Can you work these out from the model? Positions are in its coordinate system, mm. A direction names the side the tool comes from. Coordinates: 2 decimals unless noted, no trailing zeros. Order: outer loops, then holes, each group sorted by start corner. A loop starts at its lowest first (then second) coordinate and runs counter-clockwise, first axis right, second up. Notation, with made-up numbers: (-20, 87) -> (32, 87) arc R14 cw to (32, 107) -> close; hole circle Ø11 at (51.5, 18). An arc over 180 degrees is marked (long way). Write item = value, one per line. Start each with the question number.
from build123d import *

# Parameters (mm, degrees)
AXIAL_HOLES_DEPTH                            = 167.945530039
AXIAL_HOLES_DEPTH_BACK                       = 167.945530039
SKETCH2_R                                    = 2.3
SKETCH2_R_2                                  = 1.65
DRY_START                                    = 159.2
SKETCH3_W                                    = 1
SKETCH3_H                                    = 8.8
DRY_INTERFACE_VENT_NOT_A_COOLANT_PASSA_DEPTH = 0.5


with BuildPart() as part:
    # Axial profile (mm) → Full revolution (revolve)
    with BuildSketch(Plane.XY, mode=Mode.PRIVATE) as full_revolution_sk:
        Polygon((156.7, 0), (159.65, 0), (159.65, 26.2), (159.2, 26.2), (159.2, 27.2), (159.7, 27.2), (159.7, 34.4), (156.7, 34.4), align=None)
    revolve(full_revolution_sk.sketch.rotate(Axis((-110, 0, 0), (1, 0, 0)), 90), axis=Axis((-110, 0, 0), (1, 0, 0)))

    # Sketch2 → Axial holes (cut, two sides: drawn at the far end of the back side and taken through both)
    with BuildSketch(Plane(origin=(0, 0, 0), x_dir=(0, 0, -1), z_dir=(1, 0, 0)).offset(-AXIAL_HOLES_DEPTH_BACK)):
        with Locations(Location((-1.977382665, 12.848733704, 0), (0, 0, 180))):
            Circle(SKETCH2_R)
        with Locations(Location((-7.687206041, 10.483647423, 0), (0, 0, 180))):
            Circle(SKETCH2_R)
        with Locations((-29.4, 0)):
            Circle(SKETCH2_R_2)
        with Locations((14.7, -25.461146871)):
            Circle(SKETCH2_R_2)
        with Locations((14.7, 25.461146871)):
            Circle(SKETCH2_R_2)
    extrude(amount=AXIAL_HOLES_DEPTH + AXIAL_HOLES_DEPTH_BACK, mode=Mode.SUBTRACT)

    # Sketch3 → Dry interface vent - NOT a coolant passage (cut)
    with BuildSketch(Plane(origin=(0, 0, 0), x_dir=(0, 0, -1), z_dir=(1, 0, 0)).offset(DRY_START)):
        with Locations((0, 30.6)):
            Rectangle(SKETCH3_W, SKETCH3_H)
    extrude(amount=DRY_INTERFACE_VENT_NOT_A_COOLANT_PASSA_DEPTH, mode=Mode.SUBTRACT)


solid = part.part
(1) Imagine slicing it at D-D (x = 157.25). Write out the boundary of the cut face in (y, z), plus the area to 3 significant figures.
(2) Imagine slicing it at A-A (z = 2.5). Write out the boundary of the cut face in (x, y), plus the area to 3 significant figures.
(3) Imagine slicing it at B-B (y = 30). Write out the boundary of the cut face in (x, z).
(4) Imagine slicing it at C-C (z = -14.7). Write out the boundary of the cut face in (x, y), plus the area to 3 significant figures.
(5) For faces 5 (the face through (159.42, -17.71, -19.31)), 6 (the face through (158.18, -24.07, -15.59)), which set-ups out of +Z, -Z, +X, -X, +Y, -Y let a thin tool reach every point of the face, with its end or its side?
(6) For P1, Ø4.5, axis at y = 0, z = 29.4, coming from the +X side; P2, Ø6, axis at y = 10.48, z = 7.69, coming from the +X side, each with a flat end and sliding along its axis, tell me the tip position at first contact or that it passes through.
(7) If I drill on L1, parallel to Z at x = 159.3, y = 10; L2, parallel to Y at x = 159.4, z = -5.5; L3, parallel to Y at x = 159.35, z = -10.5, over which ranges is the centre line in solid material (lowest first)? Write a range as from..to.
(8) Thinking about a two-plate mould opening in Y: for faces 1 (the face through (159.7, -26, -10)), 2 (the face through (158.179, -1.513, -34.367)), 3 (the face through (158.15, 8.93, 5.99)), 4 (the face through (158.179, 0.496, 27.826)), which applies, +Y half, -Y half, draft (parallel to the pull), parting line (faces both ways), or undercut?
Result set:
q1.outline = circle Ø68.8 at (0, 0); hole circle Ø3.3 at (-25.46, -14.7); hole circle Ø3.3 at (0, 29.4); hole circle Ø4.6 at (10.48, 7.69); hole circle Ø4.6 at (12.85, 1.98); hole circle Ø3.3 at (25.46, -14.7)
q1.area = 3,660 mm2
q2.outline = (156.7, -34.31) -> (159.7, -34.31) -> (159.7, -27.08) -> (159.2, -27.08) -> (159.2, -26.08) -> (159.65, -26.08) -> (159.65, 10.61) -> (156.7, 10.61) -> close; (156.7, 15.09) -> (159.65, 15.09) -> (159.65, 26.08) -> (159.2, 26.08) -> (159.2, 27.08) -> (159.7, 27.08) -> (159.7, 34.31) -> (156.7, 34.31) -> close
q2.area = 189 mm2
q3.outline = (156.7, -16.83) -> (159.7, -16.83) -> (159.7, -0.5) -> (159.2, -0.5) -> (159.2, 0.5) -> (159.7, 0.5) -> (159.7, 16.83) -> (156.7, 16.83) -> close
q4.outline = (156.7, -31.1) -> (159.7, -31.1) -> (159.7, -27.11) -> (156.7, -27.11) -> close; (156.7, -23.81) -> (159.7, -23.81) -> (159.7, -22.89) -> (159.2, -22.89) -> (159.2, -21.69) -> (159.65, -21.69) -> (159.65, 21.69) -> (159.2, 21.69) -> (159.2, 22.89) -> (159.7, 22.89) -> (159.7, 23.81) -> (156.7, 23.81) -> close; (156.7, 27.11) -> (159.7, 27.11) -> (159.7, 31.1) -> (156.7, 31.1) -> close
q4.area = 163 mm2
q5.face_5 = +X
q5.face_6 = +X, -X
q6.P1 = 159.7
q6.P2 = 159.65
q7.L1 = -32.91..-25.3, -24.22..5.44, 9.94..24.22, 25.3..32.91
q7.L2 = -33.96..-26.64, -25.62..25.62, 26.64..33.96
q7.L3 = -32.76..-25.09, -24..24, 25.09..32.76
q8.face_1 = draft
q8.face_2 = parting line
q8.face_3 = undercut
q8.face_4 = undercut
